Part model, mm, in its own coordinate system. A direction names the side the tool comes from. Give positions to 0.01 mm unless a question says otherwise; leave off trailing zeros. Order: outer loops, then holes, each group sorted by start corner. A loop starts at its lowest first (then second) coordinate and runs counter-clockwise, first axis right, second up.
1. Probe line 1 (Y direction, x = 1.5, z = 9.5); line 2 (Z direction, x = -15.5, y = 2); line 3 (Y direction, x = 6.5, z = 14). List the from-to ranges inside material, lowest first.
2. Mould opens along X. For faces 4 (the flat face through (-39.23, -4.14, 12.32)), 5 (the flat face through (-30.878, 2.708, 12.629)), 6 (the flat face through (39.47, -1.894, 12.325)), 7 (the flat face through (-43.56, 0.61, 12.32)) say: +X half, -X half, draft (parallel to the pull), parting line (faces both ways), or undercut.
3. Slice it at A-A on x = -2.5. List the corners of the cut face in (y, z).
4. Drop flat-ended pins along their axis: pin 1 Ø2 at (x, y) = (1.5, 1) entering from +Z; pin 2 Ø1 at (x, z) = (29, 6) entering from -Y; pin 3 Ø4 at (x, z) = (-34, 21.5) entering from -Y; pin 4 Ø1 at (x, z) = (33.5, 20.5) entering from +Y. Give the stop position or say it passes through.
5. Which spindle directions (+Z, -Z, +X, -X, +Y, -Y) get a long thin tool onto all of the face, cutting with end or side? Do faces 1 (the flat face through (-21.084, 3.507, 12.629)), 2 (the flat face through (30.701, 0.702, 12.325)), 3 (the flat face through (-2.677, -0.647, 12.325)). Say none if no direction does.
6. Slice it at B-B on x = 39.5. List the corners of the cut face in (y, z), and give its area (3 significant figures).
from build123d import *

# Parameters (mm, degrees)
F1_DEPTH = 25
F2_T     = -0.6


# Not quite as in the source:
# - a feature names something its author has since deleted; it is built from what else it names


with BuildPart() as f1:
    # F0 (on Top) → F1 (new body)
    with BuildSketch(Plane.XY):
        Polygon((46.698, -2.739), (46.698, -2.206), (45.044, -1.922), (43.064, -1.555), (40.775, -1.102), (38.202, -0.597), (35.37, -0.07), (35.37, -1.473), (38.202, -1.754), (40.775, -2.038), (43.064, -2.306), (45.044, -2.543), align=None)
        Polygon((35.37, -1.473), (35.37, -0.07), (32.309, 0.453), (29.048, 0.959), (25.616, 1.44), (22.043, 1.892), (18.359, 2.315), (14.594, 2.708), (10.778, 3.069), (6.937, 3.396), (3.099, 3.68), (-0.735, 3.917), (-4.565, 4.101), (-8.362, 4.224), (-12.113, 4.281), (-15.796, 4.268), (-19.391, 4.184), (-22.88, 4.026), (-26.24, 3.795), (-29.451, 3.49), (-32.496, 3.111), (-35.352, 2.66), (-38.001, 2.139), (-40.424, 1.558), (-42.605, 0.932), (-44.532, 0.283), (-46.189, -0.373), (-47.567, -1.019), (-48.662, -1.638), (-49.452, -2.219), (-49.902, -2.749), (-50, -3.09), (-49.902, -3.383), (-49.452, -3.705), (-48.662, -3.939), (-47.567, -4.107), (-46.189, -4.221), (-44.532, -4.281), (-42.605, -4.278), (-40.424, -4.207), (-38.001, -4.067), (-35.352, -3.856), (-32.496, -3.581), (-29.451, -3.25), (-26.24, -2.88), (-22.88, -2.485), (-19.391, -2.083), (-15.796, -1.692), (-12.113, -1.33), (-8.362, -1.011), (-4.565, -0.747), (-0.735, -0.545), (3.099, -0.41), (6.937, -0.339), (10.778, -0.331), (14.594, -0.379), (18.359, -0.477), (22.043, -0.615), (25.616, -0.784), (29.048, -0.983), (32.309, -1.213), align=None)
    extrude(amount=F1_DEPTH)

    # F2
    f2_openings = [f1.faces().sort_by_distance(p)[0] for p in [
        (-12.597329, 0.423659, 25),
    ]]
    offset(amount=F2_T, openings=f2_openings)


solid = f1.part
Data:
1. line 1: y = -0.47 to 0.13, 3.18 to 3.78
1. line 2: z = 0 to 0.6
1. line 3: y = -0.35 to 0.25, 2.83 to 3.43
2. face 4: +X half
2. face 5: undercut
2. face 6: undercut
2. face 7: -X half
3. outline: (-0.64, 0) - (4, 0) - (4, 25) - (3.4, 25) - (3.4, 0.6) - (-0.04, 0.6) - (-0.04, 25) - (-0.64, 25) - close
4. pin 1: stops at z = 25
4. pin 2: stops at y = -1.01
4. pin 3: stops at y = -3.91
4. pin 4: stops at y = 0.33
5. face 1: +Z
5. face 2: +Z, -Z, +X, +Y
5. face 3: +Z, -Z, -Y
6. outline: (-1.9, 0) - (-0.85, 0) - (-0.85, 25) - (-1.9, 25) - close
6. area: 26.1 mm2
